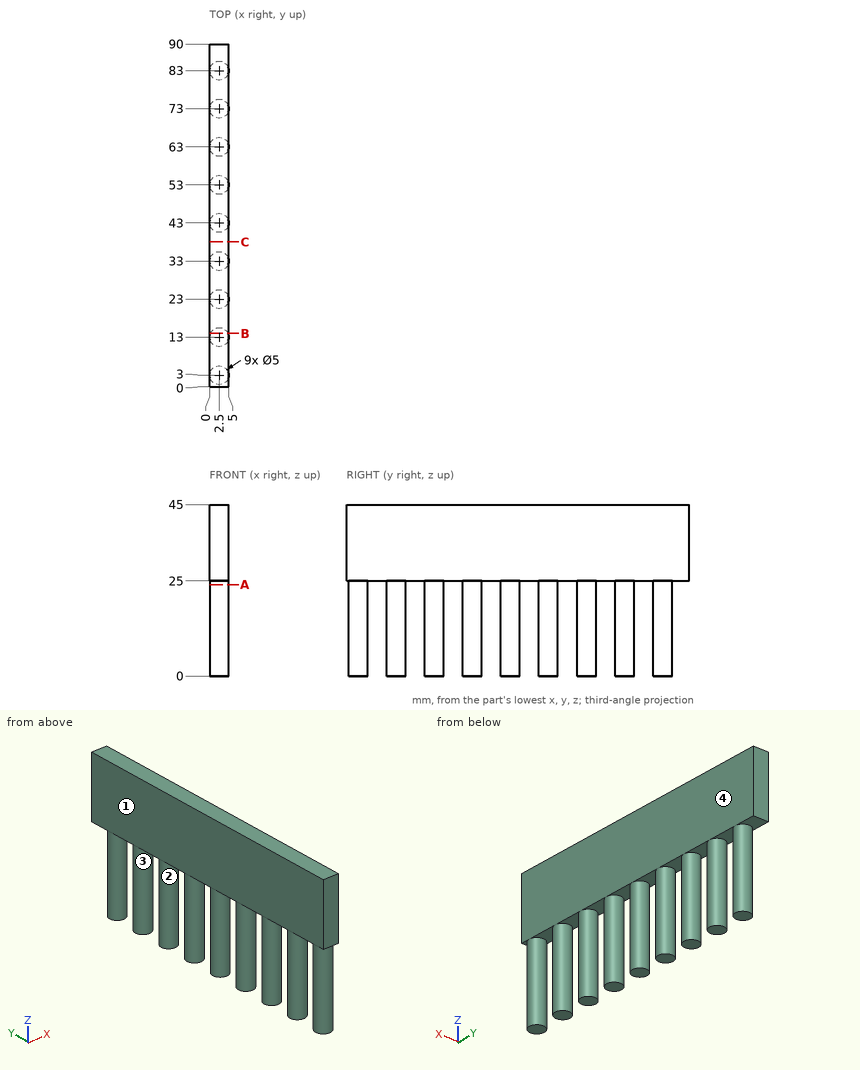
Can you work these out from the drawing? Everything is in mm from the part's minimum corner. A direction names the side the tool comes from. Coordinates: 2 decimals unless noted, no trailing zeros. Write each loop counter-clockwise with the first axis right and the second up, starting at its lowest first coordinate (ties: lowest second). Pieces come first, ordered by that corner, then holes. Notation, with made-up numbers: (-25.75, -23) - (26.25, -23) arc R20 cw to (26.25, -6) - close; hole circle Ø4 at (-5, -4). An arc over 180 degrees is marked (long way). Use a Markdown table: item, result.
Q1. Thinking about a two-plate mould opening in Y: for the marked faces 3 and 4, which applies, +Y half, -Y half, draft (parallel to the pull), parting line (faces both ways), or undercut?
Geometry check:
| item | result |
|---|---|
| face 3 | undercut |
| face 4 | draft |
Q2. Which directions (+Z, -Z, +X, -X, +Y, -Y) give clear straight access to the entire face, cutting with the end or side of a thin tool? Please do the marked faces 1 and 2.
Geometry check:
| item | result |
|---|---|
| face 1 | +Z, -Z, -X, +Y, -Y |
| face 2 | -Z |
Q3. Imagine slicing it at C-C (y = 38). List the corners of the cut face in (x, z) for me, and give its area (3 significant figures).
Geometry check:
| item | result |
|---|---|
| outline | (0, 25) - (5, 25) - (5, 45) - (0, 45) - close |
| area | 100 mm2 |
Q4. Imagine slicing it at B-B (y = 14). List the corners of the cut face in (x, z) for me, and give its area (3 significant figures).
Geometry check:
| item | result |
|---|---|
| outline | (0, 25) - (0.21, 25) - (0.21, 0) - (4.79, 0) - (4.79, 25) - (5, 25) - (5, 45) - (0, 45) - close |
| area | 215 mm2 |
Q5. Imagine slicing it at A-A (z = 24). Count the separate pieces of the cut face and the enclosed holes in it, and give its area (3 significant figures).
Geometry check:
| item | result |
|---|---|
| separate pieces | 9 |
| enclosed holes | 0 |
| area | 177 mm2 |
Q6. I'm going to push flat-ended pins straight in: pin 1 Ø1 at (y, z) = (45.5, 16.5) entering from -X; pin 2 Ø3 at (x, z) = (3, 17.5) entering from -Y; pin 3 Ø1.5 at (x, y) = (3.5, 76.5) entering from -Z. Where does each tip first touch, or does it pass through?
Geometry check:
| item | result |
|---|---|
| pin 1 | stops at x = 1 |
| pin 2 | stops at y = 0.5 |
| pin 3 | stops at z = 25 |
Q7. Please list where these lines run through material, in increasing order: L1, parallel to Z at x = 1.55, y = 17; L2, parallel to X at y = 85, z = 11.5; L3, parallel to X at y = 62, z = 24.
Geometry check:
| item | result |
|---|---|
| L1 | z = 25 to 45 |
| L2 | x = 1 to 4 |
| L3 | x = 0.21 to 4.79 |
